Check sheet for the modelled part. Datum: model origin and axes. Units: mm. Face numbers are marked on the shaded views. A direction names the side the tool comes from. Give positions to 0.01 mm unless a question says otherwise; leave off trailing zeros. Order: outer loops, then holes, each group sorted by start corner. A loop starts at its lowest first (then second) coordinate and runs counter-clockwise, first axis right, second up. Notation, with made-up numbers: (11, 40.5) -> (16, 40.5) arc R9 ccw to (16, 45.5) -> close; hole circle Ø10 at (16.25, 4.5). An arc over 180 degrees is marked (long way). Answer in a Markdown table with one row per item. Add a question column.
(1) Cross-section at A-A (x = -6). Record the cut outline in (y, z), then the cut area to 3 significant figures.
(2) Set-up check for the marked faces 4 and 5: record each of +Z, -Z, +X, -X, +Y, -Y from which the full face is reachable in a straight line by a thin tool's end or side.
(3) Thickness scan on L1, parallel to Y at x = -35, z = 9.5; L2, parallel to Y at x = 35, z = 1.2; L3, parallel to Y at x = 0.5, z = 16. Record the ranges inside material, lowest first. Write a range as [from, to].
(4) Cross-section at C-C (x = 34). Record the cut outline in (y, z), then the cut area to 3 significant figures.
(5) Cross-section at B-B (z = 10.5). State how many separate pieces and enclosed holes the cut face has, then the cut area to 3 significant figures.
(6) Go/stop test with flat-tipped pins: pin 1 (2.5 mm diameter, centred on y = 7, z = 10, fed in from +X); pin 2 (3 mm diameter, centred on x = -35, y = 25, fed in from -Z); pin 3 (6 mm diameter, centred on x = -9, y = 22.5, fed in from -Z); pin 4 (13 mm diameter, centred on x = -12, y = 3.5, fed in from -Z). Record where each tip stops, or that it passes through.
(7) Cross-section at D-D (x = 9). Record the cut outline in (y, z), then the cut area to 3 significant figures.
(8) Release check for a two-part mould opening along X. For the marked faces 1, 2 and 3 record: released by +X, released by -X, zero draft, split by the parting line, or undercut.
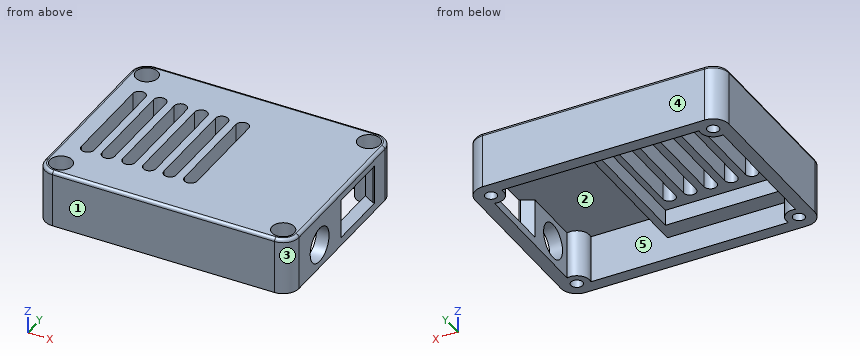
```python
from build123d import *

# Parameters (mm, degrees)
BOSS_EXTRUDE1_DEPTH = 18
CUT_EXTRUDE1_DEPTH  = 7
SKETCH3_R           = 5.5
SKETCH3_W           = 12.4
SKETCH3_H           = 19.5
CUT_EXTRUDE2_DEPTH  = 22
CUT_EXTRUDE3_DEPTH  = 8
FILLET1_R           = 1
SKETCH7_W           = 40.5
SKETCH7_H           = 40.5
CUT_EXTRUDE5_DEPTH  = 5
CUT_EXTRUDE7_DEPTH  = 52.419840529
SKETCH10_R          = 3.5
CUT_EXTRUDE8_DEPTH  = 14
SKETCH11_R          = 1.85
CUT_EXTRUDE9_DEPTH  = 52.923019943
CHAMFER1_SIZE       = 2
CHAMFER1_SIZE2      = 3.464101615


with BuildPart() as part:
    # Sketch1 → Boss-Extrude1 (new body)
    with BuildSketch(Plane.XY):
        with BuildLine():
            Line((-35, 30), (35, 30))
            ThreePointArc((35, 30), (38.535533906, 28.535533906), (40, 25))
            Line((40, 25), (40, -25))
            ThreePointArc((40, -25), (38.535533906, -28.535533906), (35, -30))
            Line((35, -30), (-35, -30))
            ThreePointArc((-35, -30), (-38.535533906, -28.535533906), (-40, -25))
            Line((-40, -25), (-40, 25))
            ThreePointArc((-40, 25), (-38.535533906, 28.535533906), (-35, 30))
        make_face()
    extrude(amount=BOSS_EXTRUDE1_DEPTH)

    # Sketch2 → Cut-Extrude1 (cut)
    with BuildSketch(Plane(origin=(0, 0, 0), x_dir=(-1, 0, 0), z_dir=(0, 0, -1))):
        with BuildLine():
            Line((-36, 21.127016654), (-36, -21.127016654))
            ThreePointArc((-36, -21.127016654), (-32.171572875, -22.171572875), (-31.127016654, -26))
            Line((-31.127016654, -26), (31.127016654, -26))
            ThreePointArc((31.127016654, -26), (32.171572875, -22.171572875), (36, -21.127016654))
            Line((36, -21.127016654), (36, 21.127016654))
            ThreePointArc((36, 21.127016654), (32.171572875, 22.171572875), (31.127016654, 26))
            Line((31.127016654, 26), (-31.127016654, 26))
            ThreePointArc((-31.127016654, 26), (-32.171572875, 22.171572875), (-36, 21.127016654))
        make_face()
    extrude(amount=-CUT_EXTRUDE1_DEPTH, mode=Mode.SUBTRACT)

    # Sketch3 → Cut-Extrude2 (cut)
    with BuildSketch(Plane(origin=(40, 0, 0), x_dir=(0, 0, -1), z_dir=(1, 0, 0))):
        with Locations(Location((-7.5, -13, 0), (0, 0, 90))):
            Circle(SKETCH3_R)
        with Locations((-8.8, 9.25)):
            Rectangle(SKETCH3_W, SKETCH3_H)
    extrude(amount=-CUT_EXTRUDE2_DEPTH, mode=Mode.SUBTRACT)

    # Sketch4 → Cut-Extrude3 (cut)
    with BuildSketch(Plane(origin=(0, 0, 7), x_dir=(-1, 0, 0), z_dir=(0, 0, -1))):
        with BuildLine():
            Line((-31.127016654, -26), (-7, -26))
            Line((-7, -26), (-7, 26))
            Line((-7, 26), (-31.127016654, 26))
            ThreePointArc((-31.127016654, 26), (-32.171572875, 22.171572875), (-36, 21.127016654))
            Line((-36, 21.127016654), (-36, -21.127016654))
            ThreePointArc((-36, -21.127016654), (-32.171572875, -22.171572875), (-31.127016654, -26))
        make_face()
    extrude(amount=-CUT_EXTRUDE3_DEPTH, mode=Mode.SUBTRACT)

    # Fillet1
    fillet1_edges = [part.edges().sort_by_distance(p)[0] for p in [
        (-38.535533906, 28.535533906, 18),
        (-40, 0, 18),
        (-38.535533906, -28.535533906, 18),
        (0, -30, 18),
        (38.535533906, -28.535533906, 18),
        (40, 0, 18),
        (38.535533906, 28.535533906, 18),
        (0, 30, 18),
    ]]
    fillet(fillet1_edges, radius=FILLET1_R)

    # Sketch7 → Cut-Extrude5 (cut)
    with BuildSketch(Plane(origin=(0, 0, 7), x_dir=(-1, 0, 0), z_dir=(0, 0, -1))):
        with Locations((15.75, 0)):
            Rectangle(SKETCH7_W, SKETCH7_H)
    extrude(amount=-CUT_EXTRUDE5_DEPTH, mode=Mode.SUBTRACT)

    # Sketch9 → Cut-Extrude7 (cut, through all)
    with BuildSketch(Plane(origin=(0, 0, 12), x_dir=(-1, 0, 0), z_dir=(0, 0, -1))):
        with BuildLine():
            Line((1.5, 15), (1.5, -15))
            ThreePointArc((1.5, -15), (-0.5, -17), (-2.5, -15))
            Line((-2.5, -15), (-2.5, 15))
            ThreePointArc((-2.5, 15), (-0.5, 17), (1.5, 15))
        make_face()
        with BuildLine():
            Line((8, 15), (8, -15))
            ThreePointArc((8, -15), (6, -17), (4, -15))
            Line((4, -15), (4, 15))
            ThreePointArc((4, 15), (6, 17), (8, 15))
        make_face()
        with BuildLine():
            Line((14.5, 15), (14.5, -15))
            ThreePointArc((14.5, -15), (12.5, -17), (10.5, -15))
            Line((10.5, -15), (10.5, 15))
            ThreePointArc((10.5, 15), (12.5, 17), (14.5, 15))
        make_face()
        with BuildLine():
            Line((21, 15), (21, -15))
            ThreePointArc((21, -15), (19, -17), (17, -15))
            Line((17, -15), (17, 15))
            ThreePointArc((17, 15), (19, 17), (21, 15))
        make_face()
        with BuildLine():
            Line((27.5, 15), (27.5, -15))
            ThreePointArc((27.5, -15), (25.5, -17), (23.5, -15))
            Line((23.5, -15), (23.5, 15))
            ThreePointArc((23.5, 15), (25.5, 17), (27.5, 15))
        make_face()
        with BuildLine():
            Line((34, 15), (34, -15))
            ThreePointArc((34, -15), (32, -17), (30, -15))
            Line((30, -15), (30, 15))
            ThreePointArc((30, 15), (32, 17), (34, 15))
        make_face()
    extrude(amount=-CUT_EXTRUDE7_DEPTH, mode=Mode.SUBTRACT)

    # Sketch10 → Cut-Extrude8 (cut)
    with BuildSketch(Plane.XY.offset(18)):
        with Locations((-35, 25)):
            Circle(SKETCH10_R)
        with Locations((-35, -25)):
            Circle(SKETCH10_R)
        with Locations((35, -25)):
            Circle(SKETCH10_R)
        with Locations((35, 25)):
            Circle(SKETCH10_R)
    extrude(amount=-CUT_EXTRUDE8_DEPTH, mode=Mode.SUBTRACT)

    # Sketch11 → Cut-Extrude9 (cut, through all)
    with BuildSketch(Plane.XY.offset(4)):
        with Locations((35, -25)):
            Circle(SKETCH11_R)
        with Locations((35, 25)):
            Circle(SKETCH11_R)
        with Locations((-35, 25)):
            Circle(SKETCH11_R)
        with Locations((-35, -25)):
            Circle(SKETCH11_R)
    extrude(amount=-CUT_EXTRUDE9_DEPTH, mode=Mode.SUBTRACT)

    # Chamfer1
    chamfer1_edges = [part.edges().sort_by_distance(p)[0] for p in [
        (36, -0.5, 8.8),
        (36, 19, 8.8),
    ]]
    chamfer1_side = [part.faces().sort_by_distance(p)[0] for p in [
        (36, -3.371364126, 6.44153534),
    ]]
    chamfer(chamfer1_edges, length=CHAMFER1_SIZE, length2=CHAMFER1_SIZE2, reference=chamfer1_side[0])


solid = part.part
```
Answer below:
| question | item | result |
|---|---|---|
| 1 | outline | (-30, 0) -> (-26, 0) -> (-26, 7) -> (-20.25, 7) -> (-20.25, 12) -> (-17, 12) -> (-17, 18) -> (-29, 18) arc R1 ccw to (-30, 17) -> close; (17, 12) -> (20.25, 12) -> (20.25, 7) -> (26, 7) -> (26, 0) -> (30, 0) -> (30, 17) arc R1 ccw to (29, 18) -> (17, 18) -> close |
| 1 | area | 309 mm² |
| 2 | face 4 | +Z, -Z, +X, -X, +Y |
| 2 | face 5 | -Z |
| 3 | L1 | y = [-30, -28.5], [-21.5, -20.25], [20.25, 21.5], [28.5, 30] |
| 3 | L2 | y = [-30, -26.85], [-23.15, -21], [21, 23.15], [26.85, 30] |
| 3 | L3 | y = [-30, -17], [17, 30] |
| 4 | outline | (-30, 0) -> (-26.56, 0) -> (-26.56, 4) -> (-28.35, 4) -> (-28.35, 18) -> (-29, 18) arc R1 ccw to (-30, 17) -> close; (-23.44, 0) -> (-21.13, 0) -> (-21.13, 15) -> (21.13, 15) -> (21.13, 0) -> (23.44, 0) -> (23.44, 4) -> (21.65, 4) -> (21.65, 18) -> (-21.65, 18) -> (-21.65, 4) -> (-23.44, 4) -> close; (26.56, 0) -> (30, 0) -> (30, 17) arc R1 ccw to (29, 18) -> (28.35, 18) -> (28.35, 4) -> (26.56, 4) -> close |
| 4 | area | 233 mm² |
| 5 | separate pieces | 2 |
| 5 | enclosed holes | 5 |
| 5 | area | 1,400 mm² |
| 6 | pin 1 | stops at x = 7 |
| 6 | pin 2 | passes through |
| 6 | pin 3 | stops at z = 7 |
| 6 | pin 4 | stops at z = 12 |
| 7 | outline | (-30, 0) -> (-26, 0) -> (-26, 15) -> (26, 15) -> (26, 0) -> (30, 0) -> (30, 17) arc R1 ccw to (29, 18) -> (-29, 18) arc R1 ccw to (-30, 17) -> close |
| 7 | area | 300 mm² |
| 8 | face 1 | zero draft |
| 8 | face 2 | undercut |
| 8 | face 3 | released by +X |
